Autodesk Inventor part; units mm, degrees
ref_plane "YZ Plane" through (0, 0, 0) normal (1, 0, 0) x (0, 1, 0)
ref_plane "XZ Plane" through (0, 0, 0) normal (0, 1, 0) x (-1, 0, 0)
ref_plane "XY Plane" through (0, 0, 0) normal (0, 0, 1) x (1, 0, 0)
sketch "Sketch1" plane through (0, 0, 0) normal (0, 0, 1) x (1, 0, 0)
  circle A0 centre (0, 0) radius 10.125
  circle A1 centre (0, 0) radius 12.125
  dimension "d0" = 20.25
  dimension "d1" = 2
extrude "Extrusion1" add sketch "Sketch1" along normal blind 4
sketch "Sketch2" plane through (0, 0, 4) normal (0, 0, 1) x (1, 0, 0)
  circle A0 centre (0, 0) radius 10.125
  line L0 (4.1136, 7.125) -> (8.2272, 0)
  line L1 (8.2272, 0) -> (4.1136, -7.125)
  line L2 (4.1136, -7.125) -> (-4.1136, -7.125)
  line L3 (-4.1136, -7.125) -> (-8.2272, 0)
  line L4 (-8.2272, 0) -> (-4.1136, 7.125)
  line L5 (-4.1136, 7.125) -> (4.1136, 7.125)
  line L6 (-16.975, 0) -> (16.975, 0)
  line L7 (0, -16.975) -> (0, 16.975)
  circle A1 centre (0, 0) radius 12.125
  point P0 (0, 7.125)
  dimension "d4" = 14.25
extrude "Extrusion2" add sketch "Sketch2" along normal blind 6 contours L6 L0 L5 L7 A0 | L6 A1 L7 A0 | A0 L7 L2 L1 L6 | A0 L7 A1 L6 | L7 L5 L4 L6 A0 | A0 L6 A1 L7 | L7 A1 L6 A0 | A0 L6 L3 L2 L7
properties part number "BatterySafetyCap"
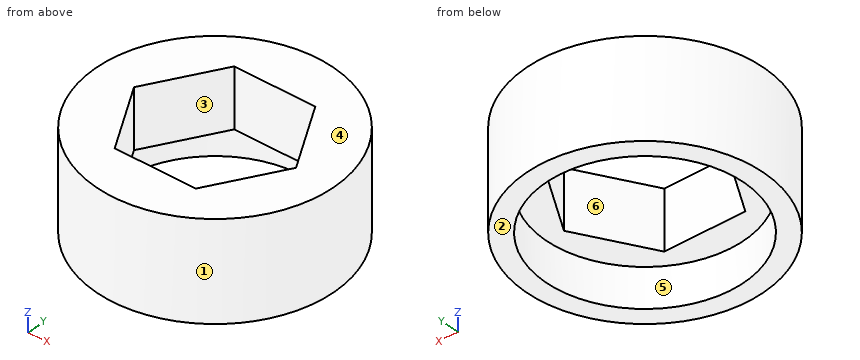
Work out the finished part from the listing and answer in its coordinate system (mm). Face numbers are marked on the shaded views. A direction names the side the tool comes from. Coordinates: 2 decimals unless noted, no trailing zeros. Write each loop counter-clockwise with the first axis right and the second up, starting at its lowest first coordinate (ties: lowest second). Pieces come first, ordered by that corner, then holes. Notation, with made-up numbers: M 77,29 L 84,29 A11 ccw 84,38 Z; hole C 9.5,8 d3. An arc over 180 degrees is marked long. Write item = value, one per line.
1. For the marked faces 4, 5 and 6, determine the directions among +Z, -Z, +X, -X, +Y, -Y from which every point of the face is accessible in a straight line to the end or side of a thin tool.
Solution:
face_4 = +Z, +X, -X, +Y, -Y
face_5 = -Z
face_6 = +Z, -Z
2. The part is cut by section A-A (z = 8.5). Determine the outline of the cut face in (x, y) (3 decimals), then the cut area to 3 significant figures.
Solution:
outline = C 0,0 d24.25; hole M -8.227,0 L -4.114,-7.125 L 4.114,-7.125 L 8.227,0 L 4.114,7.125 L -4.114,7.125 Z
area = 286 mm2
3. Flat-ended cylindrical pins translate along their axes: pin 1 (5 mm diameter, centred on y = -7.5, z = 6, fed in from -X); pin 2 (6 mm diameter, centred on x = 6, z = 5, fed in from -Y); pin 3 (5 mm diameter, centred on x = -2, y = -7, fed in from -Z). Find the tip coordinate at first contact, or state that the pin passes through.
Solution:
pin_1 = -11.05
pin_2 = -11.75
pin_3 = 4
4. The part is cut by section B-B (x = -6.75). Determine the outline of the cut face in (y, z).
Solution:
outline = M -10.07,0 L -7.55,0 L -7.55,4 L -2.56,4 L -2.56,10 L -10.07,10 Z; M 2.56,4 L 7.55,4 L 7.55,0 L 10.07,0 L 10.07,10 L 2.56,10 Z
5. The part is cut by section C-C (y = -3.75). Determine the outline of the cut face in (x, z).
Solution:
outline = M -11.53,0 L -9.4,0 L -9.4,4 L -6.06,4 L -6.06,10 L -11.53,10 Z; M 6.06,4 L 9.4,4 L 9.4,0 L 11.53,0 L 11.53,10 L 6.06,10 Z
6. Straight lines are drawn through the part: line 1 (Y direction, x = 0, z = 1.95) (3 decimals); line 2 (Z direction, x = 2.25, y = 9.5); line 3 (X direction, y = -5.5, z = 3.75). For each, find the intervals that lie inside material, in ascending order. Write a range as from..to.
Solution:
line_1 = -12.125..-10.125, 10.125..12.125
line_2 = 4..10
line_3 = -10.81..-8.5, 8.5..10.81
7. Determine the mould class of the marked faces 1, 2 and 3 for opening direction Y: released by +Y, released by -Y, zero draft, split by the parting line, or undercut.
Solution:
face_1 = split by the parting line
face_2 = zero draft
face_3 = undercut
8. The part is cut by section D-D (y = -7.75). Determine the outline of the cut face in (x, z), then the cut area to 3 significant figures.
Solution:
outline = M -9.32,0 L -6.52,0 L -6.52,4 L 6.52,4 L 6.52,0 L 9.32,0 L 9.32,10 L -9.32,10 Z
area = 134 mm2
